Verification items for this drawing (mm, ordinates from the low corner). Round coordinates to 2 decimals unless told otherwise and drop trailing zeros. Order: outer loops, then holes, each group sorted by start corner. A loop starts at its lowest first (then second) coordinate and runs counter-clockwise, first axis right, second up. Notation, with made-up numbers: (-15.75, 52.5) -> (24.25, 52.5) arc R9 ccw to (24.25, 58.5) -> close; hole circle Ø11 at (-9, 38.25). An arc over 180 degrees is marked (long way). Answer in a Markdown table with one row per item. Add a question column.
1. Draft check along Y on the marked faces 1, 2 and 3. Enter one of: +Y half, -Y half, draft (parallel to the pull), parting line (faces both ways), or undercut.
2. Sectioned sample at A-A, the plane x = 76.2. Record the boundary of the cut face in (y, z) (1 decimal), then the cut area to 3 significant figures.
3. Sectioned sample at D-D, the plane x = 22. Record the boundary of the cut face in (y, z) (1 decimal), then the cut area to 3 significant figures.
4. Sectioned sample at B-B, the plane z = 8.25. Record the boundary of the cut face in (x, y) (1 decimal), then the cut area to 3 significant figures.
5. Material ranges on L1, parallel to X at y = 14, z = 2; L2, parallel to X at y = 82, z = 7.5; L3, parallel to Y at x = 76.2, z = 8.75 (1 decimal), recorded low to high. Write a range as from..to.
6. Sectioned sample at C-C, the plane y = 39. Record the boundary of the cut face in (x, z), then the cut area to 3 significant figures.
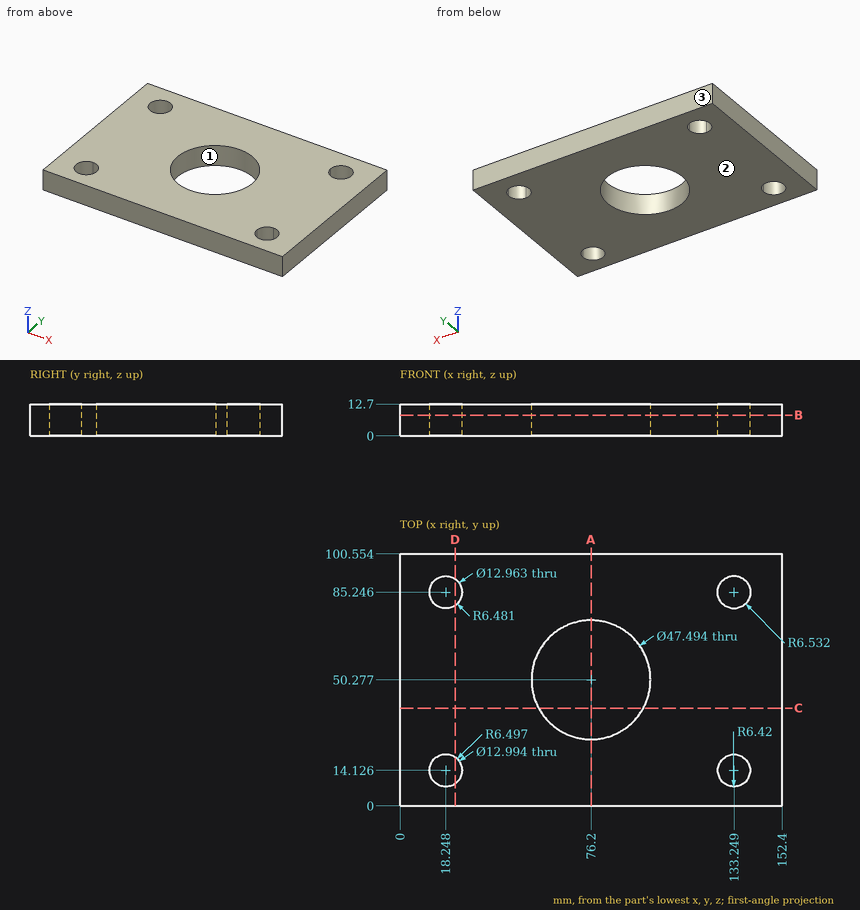
Answer key:
| question | item | result |
|---|---|---|
| 1 | face 1 | undercut |
| 1 | face 2 | draft |
| 1 | face 3 | +Y half |
| 2 | outline | (0, 0) -> (26.5, 0) -> (26.5, 12.7) -> (0, 12.7) -> close; (74, 0) -> (100.6, 0) -> (100.6, 12.7) -> (74, 12.7) -> close |
| 2 | area | 674 mm² |
| 3 | outline | (0, 0) -> (8.8, 0) -> (8.8, 12.7) -> (0, 12.7) -> close; (19.4, 0) -> (80, 0) -> (80, 12.7) -> (19.4, 12.7) -> close; (90.5, 0) -> (100.6, 0) -> (100.6, 12.7) -> (90.5, 12.7) -> close |
| 3 | area | 1,010 mm² |
| 4 | outline | (0, 0) -> (152.4, 0) -> (152.4, 100.6) -> (0, 100.6) -> close; hole circle Ø13 at (18.2, 14.1); hole circle Ø13 at (18.2, 85.2); hole circle Ø47.5 at (76.2, 50.3); hole (126.7, 85.2) arc R6.5 ccw to (133.2, 78.7) arc R6.5 ccw (long way) to start; hole (126.8, 14.1) arc R6.4 ccw (long way) to (133.2, 20.5) arc R6.4 ccw to start |
| 4 | area | 13,000 mm² |
| 5 | L1 | x = 0..11.75, 24.74..126.83, 139.67..152.4 |
| 5 | L2 | x = 0..12.64, 23.86..127.58, 138.92..152.4 |
| 5 | L3 | y = 0..26.5, 74..100.6 |
| 6 | outline | (0, 0) -> (55.3, 0) -> (55.3, 12.7) -> (0, 12.7) -> close; (97.1, 0) -> (152.4, 0) -> (152.4, 12.7) -> (97.1, 12.7) -> close |
| 6 | area | 1,400 mm² |
